```python
from build123d import *
from OCP.BRepFilletAPI import BRepFilletAPI_MakeChamfer

# Parameters (mm, degrees)
FILLET1_R           = 0.2
SKETCH2_R           = 4.9
SKETCH2_R_2         = 3.9
CUT_EXTRUDE1_DEPTH  = 0.1
SKETCH3_W           = 2
SKETCH3_H           = 0.3
SKETCH3_W_2         = 0.3
SKETCH3_H_2         = 2
EXTRUDE_THIN1_DEPTH = 3.6
CHAMFER1_SIZE       = 0.4
CHAMFER1_SIZE2      = 0.692820323
CHAMFER2_SIZE       = 3
CHAMFER2_SIZE2      = 1.091910703


with BuildPart() as part:
    # Sketch1 → Revolve1 (revolve)
    with BuildSketch(Plane(origin=(0, 0, 0), x_dir=(0, 0, -1), z_dir=(1, 0, 0))):
        Polygon((0, 1.6), (-3.9, 1.6), (-3.9, 1.5), (-5.5, 1.5), (-6.9, 0.5), (-6.9, 0), (-6, 0), (-6, -15), (-4.7, -15), (-4.7, -16.1), (0, -16.1), align=None)
    revolve(axis=Axis((0, 14.375, 0), (0, -1, 0)))

    # Fillet1
    # the kernel refuses this fillet: 0.2 mm, written as the material it takes off along each edge
    with BuildSketch(Plane(origin=(0, 1.6, 0), x_dir=(0, 0, 1), z_dir=(1, 0, 0))) as fillet1_piece_1:
        with BuildLine():
            CenterArc((3.726794919, 0.2), FILLET1_R, 270, 60)
            Line((3.9, 0.1), (3.903464102, 0.098))
            ThreePointArc((3.903464102, 0.098), (3.904, 0.05), (3.904, 0))
            Line((3.904, 0), (3.9, -0.004))
            Line((3.9, -0.004), (3.726794919, -0.004))
            Line((3.726794919, -0.004), (3.726794919, 0))
        make_face()
    revolve(axis=Axis((0, 1.6, 0), (0, -1, 0)), mode=Mode.SUBTRACT)

    # Sketch2 → Cut-Extrude1 (cut)
    with BuildSketch(Plane(origin=(0, 1.5, 0), x_dir=(1, 0, 0), z_dir=(0, 1, 0))):
        with Locations(Location((0, 0, 0), (0, 0, 270))):
            Circle(SKETCH2_R)
        with Locations(Location((0, 0, 0), (0, 0, 270))):
            Circle(SKETCH2_R_2, mode=Mode.SUBTRACT)
    extrude(amount=-CUT_EXTRUDE1_DEPTH, mode=Mode.SUBTRACT)

    # Sketch3 → Extrude-Thin1 (add)
    with BuildSketch(Plane.XZ.offset(16.1)):
        with Locations((0, 4)):
            Rectangle(SKETCH3_W, SKETCH3_H)
        with Locations((0, -4)):
            Rectangle(SKETCH3_W, SKETCH3_H)
        with Locations((-4, 0)):
            Rectangle(SKETCH3_W_2, SKETCH3_H_2)
        with Locations((4, 0)):
            Rectangle(SKETCH3_W_2, SKETCH3_H_2)
    extrude(amount=EXTRUDE_THIN1_DEPTH)

    # Chamfer1: one chamfer whose edges measure the first distance from different faces: ONE call of the kernel's chamfer builder (chamfer() names one face for all edges)
    chamfer1_edges_1 = [part.edges().sort_by_distance(p)[0] for p in [
        (1, -19.7, 4),
        (-1, -19.7, 4),
    ]]
    chamfer1_side_1 = [part.faces().sort_by_distance(p)[0] for p in [
        (0, -19.7, 4),
    ]]
    chamfer1_edges_2 = [part.edges().sort_by_distance(p)[0] for p in [
        (1, -19.7, -4),
        (-1, -19.7, -4),
    ]]
    chamfer1_side_2 = [part.faces().sort_by_distance(p)[0] for p in [
        (0, -19.7, -4),
    ]]
    chamfer1_edges_3 = [part.edges().sort_by_distance(p)[0] for p in [
        (-4, -19.7, -1),
        (-4, -19.7, 1),
    ]]
    chamfer1_side_3 = [part.faces().sort_by_distance(p)[0] for p in [
        (-4, -19.7, 0),
    ]]
    chamfer1_edges_4 = [part.edges().sort_by_distance(p)[0] for p in [
        (4, -19.7, 1),
        (4, -19.7, -1),
    ]]
    chamfer1_side_4 = [part.faces().sort_by_distance(p)[0] for p in [
        (4, -19.7, 0),
    ]]
    chamfer1 = BRepFilletAPI_MakeChamfer(part.part.solid().wrapped)
    for e in chamfer1_edges_1:
        chamfer1.Add(CHAMFER1_SIZE, CHAMFER1_SIZE2, e.wrapped, chamfer1_side_1[0].wrapped)  # the first distance lies on this face
    for e in chamfer1_edges_2:
        chamfer1.Add(CHAMFER1_SIZE, CHAMFER1_SIZE2, e.wrapped, chamfer1_side_2[0].wrapped)  # the first distance lies on this face
    for e in chamfer1_edges_3:
        chamfer1.Add(CHAMFER1_SIZE, CHAMFER1_SIZE2, e.wrapped, chamfer1_side_3[0].wrapped)  # the first distance lies on this face
    for e in chamfer1_edges_4:
        chamfer1.Add(CHAMFER1_SIZE, CHAMFER1_SIZE2, e.wrapped, chamfer1_side_4[0].wrapped)  # the first distance lies on this face
    add(Compound.cast(chamfer1.Shape()), mode=Mode.REPLACE)

    # Chamfer2
    chamfer2_edges = [part.edges().sort_by_distance(p)[0] for p in [
        (0, -15, -6),
    ]]
    chamfer2_side = [part.faces().sort_by_distance(p)[0] for p in [
        (0, -7.5, -6),
    ]]
    chamfer(chamfer2_edges, length=CHAMFER2_SIZE, length2=CHAMFER2_SIZE2, reference=chamfer2_side[0])


solid = part.part
```
Check sheet for the modelled part. Datum: model origin and axes. Units: mm. A direction names the side the tool comes from. Coordinates: 2 decimals unless noted, no trailing zeros. Write each loop counter-clockwise with the first axis right and the second up, starting at its lowest first coordinate (ties: lowest second). Pieces come first, ordered by that corner, then holes. Notation, with made-up numbers: (89, 4) - (93, 4) arc R21 cw to (93, 33) - close; hole circle Ø3 at (-36.75, 42.25). An arc over 180 degrees is marked (long way). One line per question, with ' | ' between items.
Item 1: Thickness scan on line 1 (Z direction, x = 0, y = -3.5); line 2 (Y direction, x = -3.25, z = 0.5); line 3 (Z direction, x = -2.25, y = -3.5). Record the ranges inside material, lowest first. Write a range as [from, to].
Determined:
line 1: z = [-6, 6] | line 2: y = [-16.1, 1.6] | line 3: z = [-5.56, 5.56]
Item 2: Access from +Z, -Z, +X, -X, +Y, -Y to the whole of each face (thin tool, end or side, straight path). Record for faces 1 (the face through (0, -6, -6)), 2 (the face through (1, 1.5, 5)), 3 (the face through (-3.85, -18, 0)), 4 (the face through (0, -18, -3.85)).
Determined:
face 1: -Y | face 2: +Y | face 3: +Z, -Z, -Y | face 4: +X, -X, -Y
Item 3: Mould release check, pull along X, two halves, no side actions. Record for faces 5 (the face through (-6, 0, -2)), 6 (the face through (3.85, -18, 0)), 7 (the face through (-1.49, -14.854, 4.732)): pulls with the +X half, pulls with the -X half, needs draft (parallel to the pull), parting line crosses it, or undercut.
Determined:
face 5: needs draft | face 6: undercut | face 7: parting line crosses it
Item 4: Sectioned sample at C-C on y = -1. Record the boundary of the cut face in (x, z), plus the area to 3 significant figures.
Determined:
outline: circle Ø12 at (0, 0) | area: 113 mm2
Item 5: Gauge pin test, flat ends, axial feed: P1, Ø1, axis at x = 0, y = -18.5, coming from the -Z side; P2, Ø3, axis at x = 0.5, y = -2.5, coming from the +Z side; P3, Ø1, axis at y = -18.5, z = -0.5, coming from the -X side. Record the tip position at first contact, or that the pin passes through.
Determined:
P1: stops at z = -4.15 | P2: stops at z = 6 | P3: stops at x = -4.15
